Autodesk Inventor part; units mm, degrees
ref_plane "YZ Plane" through (0, 0, 0) normal (1, 0, 0) x (0, 1, 0)
ref_plane "XZ Plane" through (0, 0, 0) normal (0, 1, 0) x (-1, 0, 0)
ref_plane "XY Plane" through (0, 0, 0) normal (0, 0, 1) x (1, 0, 0)
sketch "Sketch1" plane through (0, 0, 0) normal (0, 0, 1) x (1, 0, 0)
  line L0 (0, 0) -> (150, 0)
  line L1 (150, 0) -> (150, 91)
  line L2 (150, 91) -> (0, 91)
  line L3 (0, 91) -> (0, 0)
  dimension "d0" = 150
  dimension "d1" = 91
extrude "Extrusion1" add sketch "Sketch1" along normal blind 13
sketch "Sketch2" plane through (0, 0, 13) normal (0, 0, 1) x (1, 0, 0)
  line L0 (150, 0) -> (150, 91)
  line L1 (150, 91) -> (33, 91)
  line L2 (33, 91) -> (33, 66)
  line L3 (33, 66) -> (150, 66)
  line L4 (150, 66) -> (150, 91)
  line L5 (0, 0) -> (150, 0)
  line L6 (150, 0) -> (33, 0)
  line L7 (33, 0) -> (33, 25)
  line L8 (33, 25) -> (150, 25)
  line L9 (150, 25) -> (150, 0)
  dimension "d4" = 25
  dimension "d5" = 25
  dimension "d6" = 117
  dimension "d7" = 117
extrude "Extrusion2" cut sketch "Sketch2" against normal blind 9
sketch "Sketch3" plane through (0, 0, 0) normal (0, 0, -1) x (-1, 0, 0)
  line L0 (-150, 66) -> (-33, 66)
  line L1 (-33, 25) -> (-150, 25)
  line L2 (-33, 66) -> (-33, 91)
  line L3 (0, 91) -> (0, 0)
  line L4 (-150, 91) -> (0, 91)
  line L5 (0, 0) -> (-150, 0)
  line L6 (-33, 0) -> (-33, 25)
  line L7 (-124, 63) -> (-5, 63)
  line L8 (-5, 63) -> (-5, 28)
  line L9 (-5, 28) -> (-124, 28)
  line L10 (-124, 28) -> (-124, 63)
  line L11 (-150, 0) -> (-150, 91)
  dimension "d10" = 3
  dimension "d11" = 3
  dimension "d12" = 5
  dimension "d16" = 26
extrude "Extrusion3" cut sketch "Sketch3" against normal blind 10 contours L7 L8 L9 L10
sketch "Sketch4" plane through (0, 0, 13) normal (0, 0, 1) x (1, 0, 0)
  line L0 (150, 66) -> (126, 66)
  line L1 (126, 66) -> (126, 25)
  line L2 (126, 25) -> (150, 25)
  line L3 (150, 25) -> (150, 66)
  line L4 (33, 25) -> (150, 25)
  line L5 (150, 66) -> (33, 66)
  line L6 (150, 25) -> (150, 66)
  point P0 (0, 0)
  dimension "d17" = 24
extrude "Extrusion4" cut sketch "Sketch4" against normal blind 9
sketch "Sketch5" plane through (0, 0, 0) normal (0, 0, -1) x (-1, 0, 0)
  line L0 (-126, 66) -> (-33, 66)
  line L1 (-33, 25) -> (-126, 25)
  line L2 (-126, 66) -> (-98, 66)
  line L3 (-98, 66) -> (-98, 25)
  line L4 (-98, 25) -> (-126, 25)
  line L5 (-126, 25) -> (-126, 66)
  line L6 (-126, 25) -> (-126, 66)
  point P0 (0, 0)
  dimension "d20" = 28
extrude "Extrusion5" cut sketch "Sketch5" against normal blind 10
sketch "Sketch6" plane through (0, 0, 0) normal (0, 0, -1) x (-1, 0, 0)
  line L0 (-28, 5) -> (-5, 5)
  line L1 (-5, 5) -> (-5, 86)
  line L2 (-5, 86) -> (-28, 86)
  line L3 (-28, 86) -> (-28, 5)
  line L4 (0, 0) -> (-150, 0)
  line L5 (-150, 91) -> (0, 91)
  line L6 (0, 91) -> (0, 0)
  line L7 (-33, 0) -> (-33, 25)
  line L8 (-33, 66) -> (-33, 91)
  dimension "d23" = 5
  dimension "d24" = 5
  dimension "d25" = 5
  dimension "d26" = 5
extrude "Extrusion6" cut sketch "Sketch6" against normal blind 10
equation "\"d11\" = d10"
equation "\"d25\" = d24"
properties part number "Base" material "Stainless Steel"
Design review of the part built by this model. Coordinates are the model's own, in mm. A direction names the side the tool comes from. Give positions to 0.01 mm unless a question says otherwise; leave off trailing zeros. Loops run counter-clockwise (first coordinate to the right, second up) from the corner with the lowest first, then second, coordinate; pieces in that order, holes last. Notation, with made-up numbers: M -5,24 L 15,24 A21 ccw 15,49 Z; hole C 13.5,59.25 d3. An arc over 180 degrees is marked long. Return JSON: item names as keys, results as strings. Group by question number.
Item 1: Insertion check: pin 1 Ø1.5 at (x, z) = (86.5, 10) entering from -Y; pin 2 Ø3 at (x, y) = (115.5, 59.5) entering from -Z; pin 3 Ø3.5 at (y, z) = (55.5, 11.5) entering from +X. Each pin has a flat end and moves straight along its axis. Give the tip position at first contact, or say it passes through.
Item 2: We need section B-B (y = 31). Give the boundary of the cut face in (x, z), and give its area (3 significant figures).
Item 3: Mouldability with a two-part tool opening along Y and no side actions: class faces 1 (the flat face through (112, 66, 2)), 2 (the flat face through (59.4, 91, 3.5)), 3 (the flat face through (91, 66, 0)) as released by +Y, released by -Y, zero draft, split by the parting line, or undercut.
Item 4: For probe 1 along X at (y, z) = (10.5, 2.25); probe 2 along X at (y, z) = (18, 6); probe 3 along Y at (x, z) = (40.5, 2.5), list the stretches that pass through material, from the lowest coordinate up.
Item 5: We need section A-A (x = 107.5). Give the boundary of the cut face in (y, z).
Item 6: We need section D-D (x = 31). Give the boundary of the cut face in (y, z), and give its area (3 significant figures).
Item 7: We need section C-C (z = 1.5). Give the boundary of the cut face in (x, y).
Item 8: Tool access review of faces 4 (the flat face through (112, 25, 2)), 5 (the flat face through (69, 25, 9)), 6 (the flat face through (33, 79, 9)), 7 (the flat face through (126, 46, 12)): name each direction out of +Z, -Z, +X, -X, +Y, -Y from which nothing blocks a thin tool from reaching the whole face with its end or side.
Output:
{
 "1": {"pin 1": "stops at y = 25", "pin 2": "stops at z = 10", "pin 3": "stops at x = 126"},
 "2": {"outline": "M 0,0 L 5,0 L 5,10 L 126,10 L 126,13 L 0,13 Z; M 126,0 L 150,0 L 150,4 L 126,4 Z", "area": "524 mm^2"},
 "3": {"face 1": "undercut", "face 2": "released by +Y", "face 3": "zero draft"},
 "4": {"probe 1": "x = 0 to 5, 28 to 150", "probe 2": "x = 0 to 5, 28 to 33", "probe 3": "y = 0 to 28, 63 to 91"},
 "5": {"outline": "M 0,0 L 25,0 L 25,4 L 0,4 Z; M 25,10 L 66,10 L 66,13 L 25,13 Z; M 66,0 L 91,0 L 91,4 L 66,4 Z"},
 "6": {"outline": "M 0,0 L 28,0 L 28,10 L 63,10 L 63,0 L 91,0 L 91,13 L 0,13 Z", "area": "833 mm^2"},
 "7": {"outline": "M 0,0 L 150,0 L 150,91 L 0,91 Z; hole M 5,5 L 28,5 L 28,28 L 98,28 L 98,25 L 126,25 L 126,66 L 98,66 L 98,63 L 28,63 L 28,86 L 5,86 Z"},
 "8": {"face 4": "-Z", "face 5": "+Z, +X, -Y", "face 6": "+Z, +X, +Y", "face 7": "+Z, +X, +Y, -Y"}
}
